Check sheet for the modelled part. Datum: model origin and axes. Units: mm. Face numbers are marked on the shaded views. A direction names the side the tool comes from. Round coordinates to 2 decimals unless told otherwise and drop trailing zeros. Order: outer loops, then holes, each group sorted by start corner. A loop starts at its lowest first (then second) coordinate and runs counter-clockwise, first axis right, second up.
```python
from build123d import *

# Parameters (mm, degrees)
F0_R     = 38.1
F0_R_2   = 19.05
F1_DEPTH = 25.4
F2_R     = 31.75
F2_R_2   = 22.225
F3_DEPTH = 3.175
F4_R     = 31.75
F4_R_2   = 22.225
F5_DEPTH = 3.175
F6_R     = 1.905


with BuildPart() as f1:
    # F0 (on Top) → F1 (new body)
    with BuildSketch(Plane.XY):
        Circle(F0_R)
        Circle(F0_R_2, mode=Mode.SUBTRACT)
    extrude(amount=F1_DEPTH)

    # F2 (on face) → F3 (cut)
    with BuildSketch(Plane(origin=(0, 0, 0), x_dir=(1, 0, 0), z_dir=(0, 0, -1))):
        Circle(F2_R)
        Circle(F2_R_2, mode=Mode.SUBTRACT)
    extrude(amount=-F3_DEPTH, mode=Mode.SUBTRACT)

    # F4 (on face) → F5 (cut)
    with BuildSketch(Plane.XY.offset(25.4)):
        Circle(F4_R)
        Circle(F4_R_2, mode=Mode.SUBTRACT)
    extrude(amount=-F5_DEPTH, mode=Mode.SUBTRACT)

    # F6
    f6_edges = [f1.edges().sort_by_distance(p)[0] for p in [
        (-38.1, 0, 0),
        (-38.1, 0, 25.4),
        (-19.05, 0, 0),
        (-19.05, 0, 25.4),
    ]]
    fillet(f6_edges, radius=F6_R)


solid = f1.part
```
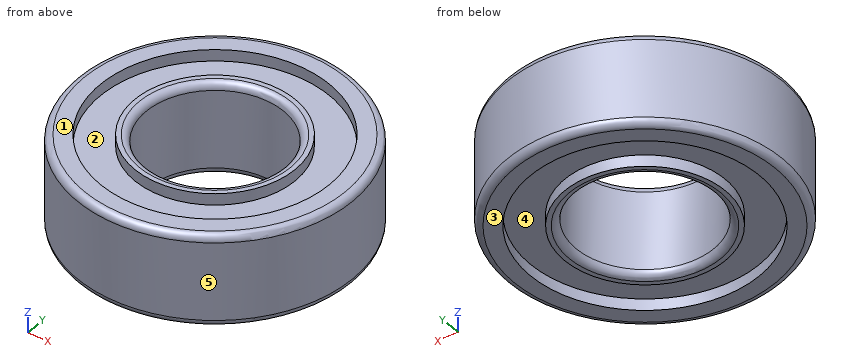
Item 1: Access from +Z, -Z, +X, -X, +Y, -Y to the whole of each face (thin tool, end or side, straight path). Record for the marked faces 1 and 2.
Answer:
face 1: +Z, +X, -X, +Y, -Y
face 2: +Z
Item 2: Go/stop test with flat-tipped pins: P1, Ø5, axis at x = -30, y = 22.5, coming from the +Z side; P2, Ø1.5, axis at x = -20.5, z = 9.5, coming from the -Y side; P3, Ø10, axis at x = 8.5, z = 16.5, coming from the +Y side; P4, Ø1, axis at x = 9, y = 16.5, coming from the -Z side. Record where each tip stops, or that it passes through.
Answer:
P1: stops at z = 25.4
P2: stops at y = -32.58
P3: stops at y = 37.94
P4: stops at z = 0.97
Item 3: Release check for a two-part mould opening along X. For the marked faces 3, 4 and 5 record: released by +X, released by -X, zero draft, split by the parting line, or undercut.
Answer:
face 3: zero draft
face 4: undercut
face 5: split by the parting line
Item 4: Sectioned sample at C-C (z = 10.5). Record the cut outline in (x, y).
Answer:
outline: circle Ø76.2 at (0, 0); hole circle Ø38.1 at (0, 0)
Item 5: Scan lines: line 1 along Y through (x, z) = (0, 23.1) (3 decimals); line 2 along Y through (x, z) = (0, 23.65) (3 decimals); line 3 along Y through (x, z) = (0, 14.5). Record each from-to range of solid material in increasing order.
Answer:
line 1: y = -38.1 to -31.75, -22.225 to -19.05, 19.05 to 22.225, 31.75 to 38.1
line 2: y = -38.094 to -31.75, -22.225 to -19.056, 19.056 to 22.225, 31.75 to 38.094
line 3: y = -38.1 to -19.05, 19.05 to 38.1
